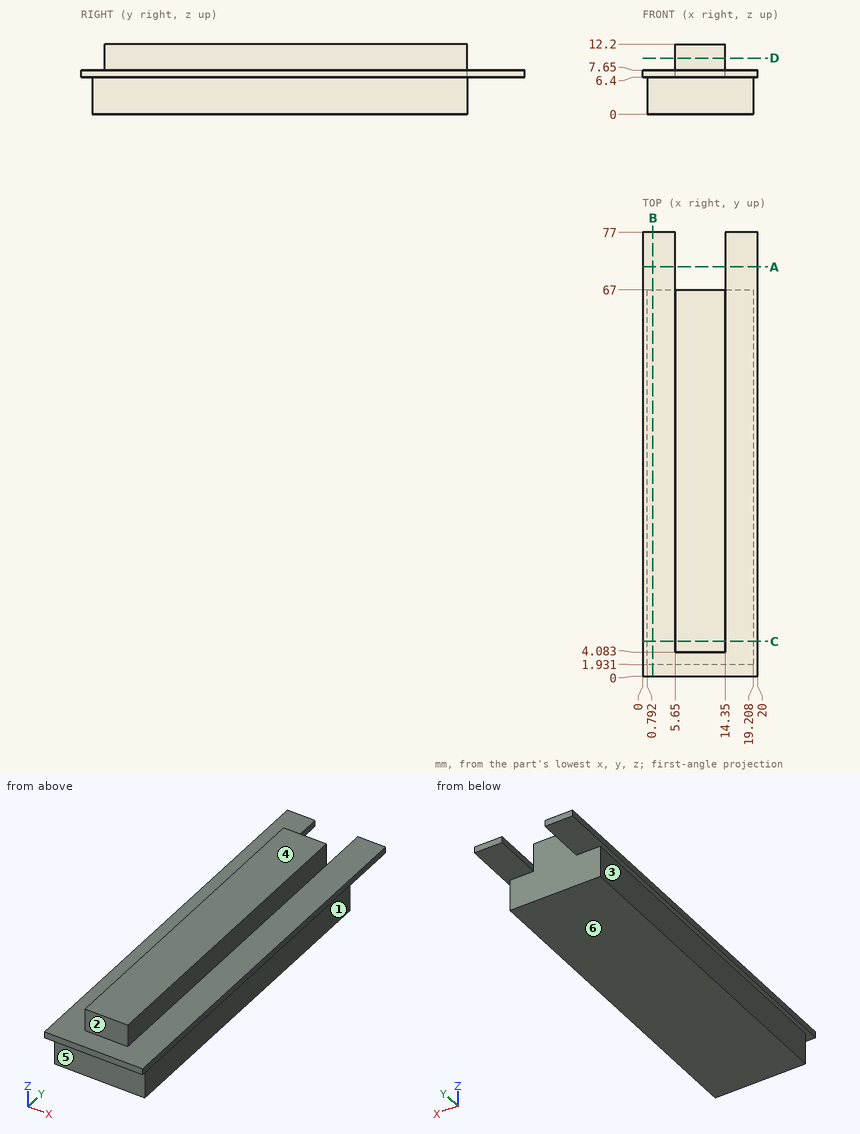
Verification items for this drawing (mm, ordinates from the low corner). A direction names the side the tool comes from. Give positions to 0.01 mm unless a question says otherwise; leave off trailing zeros. Order: outer loops, then holes, each group sorted by start corner. A loop starts at its lowest first (then second) coordinate and runs counter-clockwise, first axis right, second up.
1) Draft check along Z on the marked faces 4, 5 and 6. Enter one of: released by +Z, released by -Z, zero draft, split by the parting line, or undercut.
Results are:
face 4: released by +Z
face 5: zero draft
face 6: released by -Z
2) Cross-section at D-D (z = 9.75). Record the boundary of the cut face in (x, y), then the cut area to 3 significant figures.
Results are:
outline: (5.65, 4.08) - (14.35, 4.08) - (14.35, 67) - (5.65, 67) - close
area: 547 mm2
3) Cross-section at C-C (y = 6). Record the boundary of the cut face in (x, z), then the cut area to 3 significant figures.
Results are:
outline: (0, 6.4) - (0.79, 6.4) - (0.79, 0) - (19.21, 0) - (19.21, 6.4) - (20, 6.4) - (20, 7.65) - (14.35, 7.65) - (14.35, 12.2) - (5.65, 12.2) - (5.65, 7.65) - (0, 7.65) - close
area: 182 mm2
4) Gauge pin test, flat ends, axial feed: pin 1 (5 mm diameter, centred on y = 45, z = 3.5, fed in from +X); pin 2 (3.5 mm diameter, centred on y = 32.5, z = 10, fed in from +X); pin 3 (6 mm diameter, centred on x = 12, z = 3.5, fed in from +Y). Record the tip position at first contact, or that the pin passes through.
Results are:
pin 1: stops at x = 19.21
pin 2: stops at x = 14.35
pin 3: stops at y = 67
5) Cross-section at B-B (x = 1.75). Record the boundary of the cut face in (y, z).
Results are:
outline: (0, 6.4) - (1.93, 6.4) - (1.93, 0) - (67, 0) - (67, 6.4) - (77, 6.4) - (77, 7.65) - (0, 7.65) - close
6) Tool access check on the marked faces 1, 2 and 3. Record the directions out of +Z, -Z, +X, -X, +Y, -Y that give a thin tool (end or side, any length) a straight path to the whole face; none if there is none.
Results are:
face 1: -Z, +X, +Y, -Y
face 2: +Z, +X, -X, -Y
face 3: -Z, -X, +Y, -Y
7) Cross-section at A-A (y = 71). Record the boundary of the cut face in (x, z), then the cut area to 3 significant figures.
Results are:
outline: (0, 6.4) - (5.65, 6.4) - (5.65, 7.65) - (0, 7.65) - close; (14.35, 6.4) - (20, 6.4) - (20, 7.65) - (14.35, 7.65) - close
area: 14.1 mm2
8) Material ranges on probe 1 along Z at (x, y) = (17.75, 15.5); probe 2 along X at (y, z) = (37, 5.25); probe 3 along X at (y, z) = (45.5, 9.25), recorded low to high.
Results are:
probe 1: z = 0 to 7.65
probe 2: x = 0.79 to 19.21
probe 3: x = 5.65 to 14.35
